Can you work these out from the model? Positions are in its coordinate system, mm. Round coordinates to 2 decimals unless told otherwise and drop trailing zeros. Write each loop counter-clockwise with the first axis right and the second up, starting at its lowest first coordinate (ties: lowest second). Pieces come first, ordered by that corner, then holes. Notation, with made-up numbers: M -35.75,26 L -14.75,26 A8 cw -14.75,39 Z; hole C 27,70.5 d1. An arc over 180 degrees is marked long. Answer as a JSON object with one key per item and string values. Group by question number.
1) If we mould it in two halves opening along X, with no side actions, what happens to faces 1 (the cylindrical face through (-2.44, 26.2, 0.76)), 2 (the cylindrical face through (-44, 26, 1)), 3 (the cylindrical face through (-7.85, -8.43, 0.74))? For each: +X half, -X half, draft (parallel to the pull), parting line (faces both ways), or undercut.
2) Suppose I cut it at C-C, the plane z = 0.7. Write out the boundary of the cut face in (x, y), and give its area (3 significant figures).
3) Suppose I cut it at A-A, the plane x = -17.5. Write out the boundary of the cut face in (y, z), and give its area (3 significant figures).
4) Suppose I cut it at B-B, the plane y = 2. Write out the boundary of the cut face in (x, z), and give its area (3 significant figures).
5) Please list where these lines run through material, in increasing order: L1, parallel to X at y = 21, z = 1.35; L2, parallel to Y at x = -23, z = 0.8; L3, parallel to Y at x = -40, z = 1.2. Write a range as [from, to].
from build123d import *

# Parameters (mm, degrees)
SKETCH_1_W      = 42
SKETCH_1_H      = 42
SKETCH_1_R      = 1.6
SKETCH_1_R_2    = 11.5
EXTRUDE_1_DEPTH = 1.5
FILLET_1_R      = 1


with BuildPart() as part:
    # 草图1 → 凸台-拉伸1 (new body)
    with BuildSketch(Plane.XY):
        with Locations((-23.141791045, 5.485074627)):
            Rectangle(SKETCH_1_W, SKETCH_1_H)
        with Locations((-38.641791045, 20.985074627)):
            Circle(SKETCH_1_R, mode=Mode.SUBTRACT)
        with Locations((-23.141791045, 5.485074627)):
            Circle(SKETCH_1_R_2, mode=Mode.SUBTRACT)
        with Locations(Location((-7.641791045, 20.985074627, 0), (0, 0, 180))):
            Circle(SKETCH_1_R, mode=Mode.SUBTRACT)
        with Locations((-7.641791045, -10.014925373)):
            Circle(SKETCH_1_R, mode=Mode.SUBTRACT)
        with Locations(Location((-38.641791045, -10.014925373, 0), (0, 0, 180))):
            Circle(SKETCH_1_R, mode=Mode.SUBTRACT)
    extrude(amount=EXTRUDE_1_DEPTH)

    # 圆角1
    fillet_1_edges = [part.edges().sort_by_distance(p)[0] for p in [
        (-44.141791045, 26.485074627, 0.75),
        (-2.141791045, 26.485074627, 0.75),
        (-2.141791045, -15.514925373, 0.75),
        (-44.141791045, -15.514925373, 0.75),
    ]]
    fillet(fillet_1_edges, radius=FILLET_1_R)


solid = part.part
Results:
{
 "1": {"face 1": "+X half", "face 2": "-X half", "face 3": "undercut"},
 "2": {"outline": "M -44.14,-14.51 A1 ccw -43.14,-15.51 L -3.14,-15.51 A1 ccw -2.14,-14.51 L -2.14,25.49 A1 ccw -3.14,26.49 L -43.14,26.49 A1 ccw -44.14,25.49 Z; hole C -38.64,-10.01 d3.2; hole C -38.64,20.99 d3.2; hole C -23.14,5.49 d23; hole C -7.64,-10.01 d3.2; hole C -7.64,20.99 d3.2", "area": "1,320 mm^2"},
 "3": {"outline": "M -15.51,0 L -4.54,0 L -4.54,1.5 L -15.51,1.5 Z; M 15.51,0 L 26.49,0 L 26.49,1.5 L 15.51,1.5 Z", "area": "32.9 mm^2"},
 "4": {"outline": "M -44.14,0 L -34.1,0 L -34.1,1.5 L -44.14,1.5 Z; M -12.18,0 L -2.14,0 L -2.14,1.5 L -12.18,1.5 Z", "area": "30.1 mm^2"},
 "5": {"L1": "[-44.14, -40.24], [-37.04, -9.24], [-6.04, -2.14]", "L2": "[-15.51, -6.01], [16.98, 26.49]", "L3": "[-15.51, -10.86], [-9.17, 20.14], [21.83, 26.49]"}
}
